```python
from build123d import *

# Parameters (mm, degrees)
F0_R     = 9.525
F1_DEPTH = 25.4
F2_R     = 5.08
F3_R     = 5.08
F5_DEPTH = 11.2014


with BuildPart() as f1:
    # F0 (on Top) → F1 (new body)
    with BuildSketch(Plane.XY):
        with BuildLine():
            Line((15.347393, 38.231497), (-6.205886, 24.045919))
            Line((-6.205886, 24.045919), (-30.007427, 24.045919))
            ThreePointArc((-30.007427, 24.045919), (-35.477162, 20.92152), (-35.564335, 14.622928))
            Line((-35.564335, 14.622928), (-24.045919, -6.205886))
            Line((-24.045919, -6.205886), (-24.045919, -30.007427))
            ThreePointArc((-24.045919, -30.007427), (-20.92152, -35.477162), (-14.622928, -35.564335))
            Line((-14.622928, -35.564335), (6.205886, -24.045919))
            Line((6.205886, -24.045919), (30.007427, -24.045919))
            ThreePointArc((30.007427, -24.045919), (35.477162, -20.92152), (35.564335, -14.622928))
            Line((35.564335, -14.622928), (24.045919, 6.205886))
            Line((24.045919, 6.205886), (25.182596, 32.654602))
            ThreePointArc((25.182596, 32.654602), (21.970617, 38.451023), (15.347393, 38.231497))
        make_face()
        Circle(F0_R, mode=Mode.SUBTRACT)
    extrude(amount=F1_DEPTH)

    # F2
    f2_edges = [f1.edges().sort_by_distance(p)[0] for p in [
        (-29.805127, 4.208521, 0),
        (4.570753, 31.138708, 0),
    ]]
    fillet(f2_edges, radius=F2_R)

    # F3
    f3_edges = [f1.edges().sort_by_distance(p)[0] for p in [
        (-24.045919, -18.106656, 0),
        (4.570753, 31.138708, 25.4),
        (-18.106656, 24.045919, 25.4),
        (-24.045919, -18.106656, 25.4),
        (18.106656, -24.045919, 25.4),
        (18.106656, -24.045919, 0),
    ]]
    fillet(f3_edges, radius=F3_R)

    # F4 (on face) → F5 (cut)
    with BuildSketch(Plane.XY.offset(25.4)):
        Polygon((-5.572585, -9.652), (5.572585, -9.652), (11.14517, 0), (5.572585, 9.652), (-5.572585, 9.652), (-11.14517, 0), align=None)
    extrude(amount=-F5_DEPTH, mode=Mode.SUBTRACT)


solid = f1.part
```
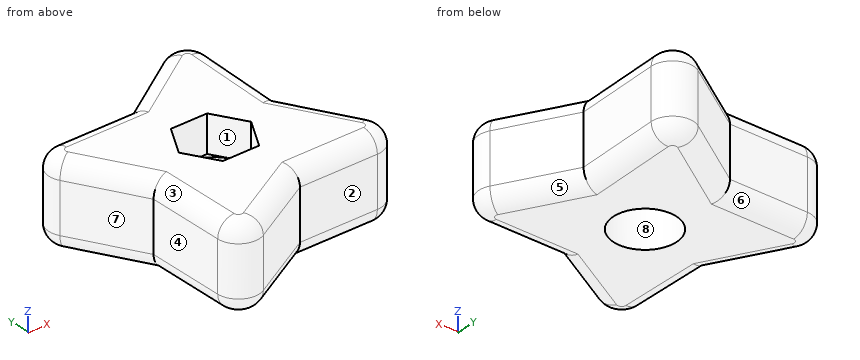
Design review of the part built by this model. Coordinates are the model's own, in mm. Face numbers are marked on the shaded views. A direction names the side the tool comes from. Round coordinates to 2 decimals unless told otherwise and drop trailing zeros. Order: outer loops, then holes, each group sorted by start corner. A loop starts at its lowest first (then second) coordinate and runs counter-clockwise, first axis right, second up. Notation, with made-up numbers: (54.25, -17) - (92.25, -17) arc R25 cw to (92.25, 1) - close; hole circle Ø10 at (21.25, 12.25). An arc over 180 degrees is marked (long way). Return JSON: item names as keys, results as strings.
Q1. The part is to be moulded in two halves that separate along X. For the marked faces 5, 6, 7 and 8, say which applies: pulls with the +X half, pulls with the -X half, needs draft (parallel to the pull), parting line crosses it, or undercut.
Computed values:
{"face 5": "pulls with the +X half", "face 6": "needs draft", "face 7": "pulls with the -X half", "face 8": "undercut"}
Q2. Consider section B-B on z = 18.25. Write out the cut boundary in (x, y), plus the area to 3 significant figures.
Computed values:
{"outline": "(-35.56, 14.62) - (-24.05, -6.21) - (-24.05, -30.01) arc R6.35 ccw to (-14.62, -35.56) - (6.21, -24.05) - (30.01, -24.05) arc R6.35 ccw to (35.56, -14.62) - (24.05, 6.21) - (25.18, 32.65) arc R6.35 ccw to (15.35, 38.23) - (-6.21, 24.05) - (-30.01, 24.05) arc R6.35 ccw to start; hole (-11.15, 0) - (-5.57, -9.65) - (5.57, -9.65) - (11.15, 0) - (5.57, 9.65) - (-5.57, 9.65) - close", "area": "2,970 mm2"}
Q3. Wall thickness on L1, parallel to Z at x = 3, y = 24.5; L2, parallel to X at y = 5, z = 16; L3, parallel to Y at x = 0, z = 5.5 (3 decimals): over which ranges is each line inside the solid? List them lowest first. Write a range as [from, to].
Computed values:
{"L1": "z = [0.02, 25.38]", "L2": "x = [-30.24, -8.26], [8.26, 24.71]", "L3": "y = [-27.478, -9.525], [9.525, 28.13]"}
Q4. Machinability: for the marked faces 1, 2, 3 and 4, which of the approach directions +Z, -Z, +X, -X, +Y, -Y give a long, thin tool a straight path to every point of the face, cutting with its end or side? Answer none if there is none.
Computed values:
{"face 1": "+Z", "face 2": "+Z, -Z, +X, -Y", "face 3": "+Z, -X, -Y", "face 4": "+Z, -Z, -X, -Y"}
Q5. For pin 1 Ø1 at (x, z) = (29, 16.5) entering from +Y; pin 2 Ø1 at (y, z) = (2, 12.5) entering from +X; pin 3 Ø4 at (x, z) = (10.5, 6) entering from -Y; pin 4 Ø22 at (x, y) = (0, 0) entering from -Z, all flat-tipped, find the tip position at first contact; note any pin that passes through.
Computed values:
{"pin 1": "stops at y = -1.85", "pin 2": "stops at x = 26.65", "pin 3": "stops at y = -24.05", "pin 4": "stops at z = 0"}
